Could you check a few things on this model? Use its own coordinates, in mm. A direction names the side the tool comes from. Round coordinates to 2 decimals unless told otherwise and drop trailing zeros. Order: outer loops, then holes, each group sorted by start corner. A loop starts at its lowest first (then second) coordinate and runs counter-clockwise, first axis right, second up. Notation, with made-up numbers: M 57,-14 L 83,-14 A10 ccw 83,-5 Z; hole C 49.25,-24 d10. An arc over 180 degrees is marked long. Write each question's results on one line, items separated by ' | '. Start each with the question number.
1. Please list where these lines run through material, in increasing order: L1, parallel to Y at x = 3.55, z = 2.45; L2, parallel to X at y = 10.75, z = 1; L3, parallel to X at y = 16.5, z = 3.5.
2. Suppose I cut it at B-B on x = 3.5. Write out the boundary of the cut face in (y, z).
3. I'm going to push flat-ended pins straight in: pin 1 (2 mm diameter, centred on x = 28, z = 2.5, fed in from +Y); pin 2 (1 mm diameter, centred on y = 8, z = 5, fed in from +X); pin 3 (1.5 mm diameter, centred on x = 8, z = 2.5, fed in from -Y); pin 4 (1.2 mm diameter, centred on y = 15.5, z = 4, fed in from +X). Where does each tip first touch, or does it pass through?
4. Suppose I cut it at A-A on z = 4.5. Write out the boundary of the cut face in (x, y), and give its area (3 significant figures).
5. We'd pull the mould along Y, two halves only. Please class faces 1 (the flat face through (18, 9, 6.9)), 2 (the flat face through (5.815, 9.965, 4.168)), 3 (the cylindrical face through (18.44, 8.52, 3.13)), 4 (the flat face through (7, 4, 3)): released by +Y, released by -Y, zero draft, split by the parting line, or undercut.
6. Suppose I cut it at C-C on y = 15.5. Write out the boundary of the cut face in (x, z).
7. For faces 5 (the flat face through (6.39, 7.36, 3.4)), 6 (the flat face through (21.876, 11, 2)), 7 (the cylindrical face through (2.965, 9.047, 2.75)), 8 (the flat face through (4, 16, 3)), 9 (the flat face through (2, 0, 3)), which set-ups out of +Z, -Z, +X, -X, +Y, -Y let a thin tool reach every point of the face, with its end or its side?
from build123d import *

# Parameters (mm, degrees)
SKETCH1_R                      = 1.5
BOSS_EXTRUDE1_DEPTH            = 6.9
CUT_EXTRUDE2_DEPTH             = 4.9
SKETCH5_R                      = 1
CUT_EXTRUDE3_DEPTH             = 7
CUT_EXTRUDE4_REACH             = 37.751
SKETCH6_R                      = 1
CUT_EXTRUDE4_DIRECTION_2_DEPTH = 2


with BuildPart() as part:
    # Sketch1 → Boss-Extrude1 (new body)
    with BuildSketch(Plane.XY):
        with BuildLine():
            Line((0, 0), (0, 18.000341084))
            Line((0, 18.000341084), (4, 18.000341084))
            Line((4, 18.000341084), (4, 14.000341084))
            Line((4, 14.000341084), (9.631516349, 14.000341084))
            Line((9.631516349, 14.000341084), (9.631516349, 18.000341084))
            Line((9.631516349, 18.000341084), (28.621516349, 18.000341084))
            ThreePointArc((28.621516349, 18.000341084), (35.324106187, 12.010882781), (30.123176491, 4.679535592))
            Line((30.123176491, 4.679535592), (9.631516349, 0))
            Line((9.631516349, 0), (9.631516349, 4))
            Line((9.631516349, 4), (4, 4))
            Line((4, 4), (4, 0))
            Line((4, 0), (0, 0))
        make_face()
        with Locations(Location((28.621516349, 11.255296941, 0), (0, 0, 180))):
            Circle(SKETCH1_R, mode=Mode.SUBTRACT)
        Polygon((14.250450019, 5.974769403), (15.118690908, 10.898808168), (13.149075402, 11.246104524), (12.280834513, 6.322065759), align=None, mode=Mode.SUBTRACT)
        Polygon((6.255421131, 12.461641767), (8.225036637, 12.114345412), (7.356795748, 7.190306647), (5.387180242, 7.537603002), align=None, mode=Mode.SUBTRACT)
    extrude(amount=BOSS_EXTRUDE1_DEPTH)

    # Sketch4 → Cut-Extrude2 (cut)
    with BuildSketch(Plane.XY):
        with BuildLine():
            Line((21.876472206, 2.796294022), (30.123176491, 4.679535592))
            ThreePointArc((30.123176491, 4.679535592), (35.324106187, 12.010882781), (28.621516349, 18.000341084))
            Line((28.621516349, 18.000341084), (21.876472206, 18.000341084))
            Line((21.876472206, 18.000341084), (21.876472206, 2.796294022))
        make_face()
    extrude(amount=CUT_EXTRUDE2_DEPTH, mode=Mode.SUBTRACT)

    # Sketch5 → Cut-Extrude3 (cut)
    with BuildSketch(Plane.ZY):
        with Locations(Location((2.45, 10.000341084, 0), (0, 0, 270))):
            Circle(SKETCH5_R)
    extrude(amount=-CUT_EXTRUDE3_DEPTH, mode=Mode.SUBTRACT)

    # Cut-Extrude4: up to this plane
    cut_extrude4_end = Plane(origin=(21.876472206, 18.000341084, 4.9), z_dir=(1, 0, 0))
    # Sketch6 → Cut-Extrude4 (cut, up to the surface)
    with BuildSketch(Plane(origin=(5.905346358, -1.041271893, 0), x_dir=(0, 0, 1), z_dir=(-0.984807753012208, 0.17364817766693114, 0)), mode=Mode.PRIVATE) as cut_extrude4_sk1:
        with Locations(Location((2.45, 10.858563908, 0), (0, 0, 270))):
            Circle(SKETCH6_R)
    cut_extrude4_tool1 = split(extrude(cut_extrude4_sk1.sketch, amount=-CUT_EXTRUDE4_REACH, mode=Mode.PRIVATE), bisect_by=cut_extrude4_end, keep=Keep.BOTH, mode=Mode.PRIVATE)
    add(cut_extrude4_tool1.solids().sort_by_distance((7.790916, 9.652326, 2.45))[0], mode=Mode.SUBTRACT)

    # Sketch6 → Cut-Extrude4 direction 2 (cut)
    with BuildSketch(Plane(origin=(5.905346358, -1.041271893, 0), x_dir=(0, 0, 1), z_dir=(-0.984807753012208, 0.17364817766693114, 0))):
        with Locations(Location((2.45, 10.858563908, 0), (0, 0, 270))):
            Circle(SKETCH6_R)
    extrude(amount=CUT_EXTRUDE4_DIRECTION_2_DEPTH, mode=Mode.SUBTRACT)


solid = part.part
Filled sheet:
1) L1: y = 0 to 9, 11 to 18 | L2: x = 0 to 5.95, 7.98 to 13.06, 15.09 to 21.88 | L3: x = 0 to 4, 9.63 to 21.88
2) outline: M 0,0 L 18,0 L 18,6.9 L 0,6.9 Z; hole C 10,2.45 d2
3) pin 1: passes through | pin 2: stops at x = 34.78 | pin 3: stops at y = 4 | pin 4: stops at x = 21.88
4) outline: M 0,0 L 4,0 L 4,4 L 9.63,4 L 9.63,0 L 21.88,2.8 L 21.88,18 L 9.63,18 L 9.63,14 L 4,14 L 4,18 L 0,18 Z; hole M 5.39,7.54 L 7.36,7.19 L 8.23,12.11 L 6.26,12.46 Z; hole M 12.28,6.32 L 14.25,5.97 L 15.12,10.9 L 13.15,11.25 Z | area: 312 mm^2
5) face 1: zero draft | face 2: undercut | face 3: undercut | face 4: released by -Y
6) outline: M 0,0 L 4,0 L 4,6.9 L 0,6.9 Z; M 9.63,0 L 21.88,0 L 21.88,4.9 L 33.86,4.9 L 33.86,6.9 L 9.63,6.9 Z
7) face 5: +Z, -Z | face 6: -Z, +X, +Y, -Y | face 7: -X | face 8: +Z, -Z, +Y | face 9: +Z, -Z, +X, -X, -Y
